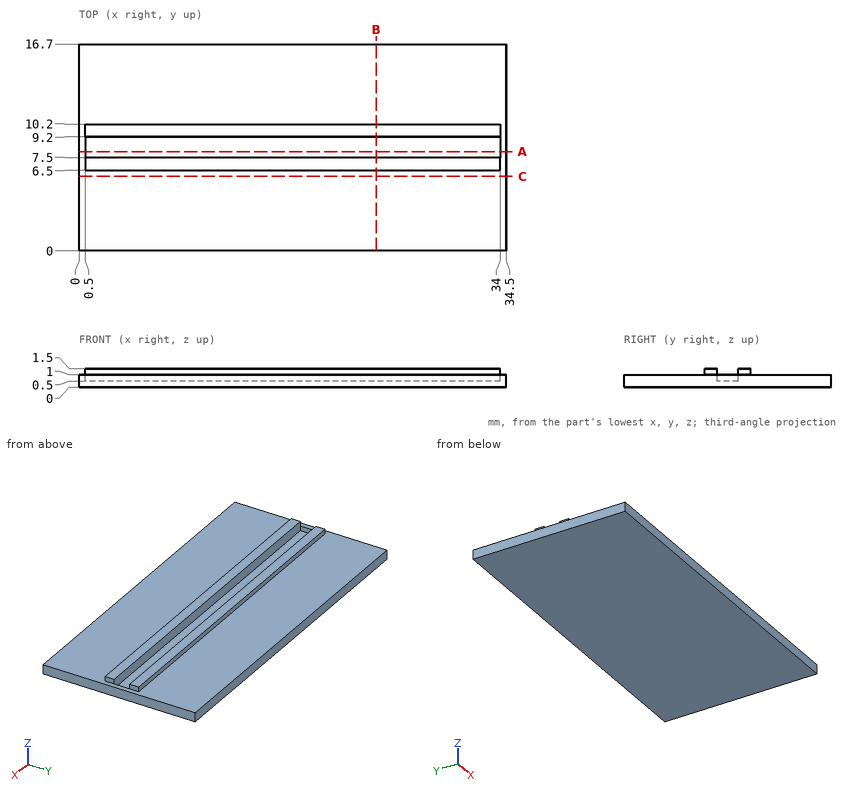
Geometry: see drawing. Coordinates: mm, zero at the bounding-box minimum. Coordinates: 2 decimals unless noted, no trailing zeros. Loops run counter-clockwise (first coordinate to the right, second up) from the corner with the lowest first, then second, coordinate; pieces in that order, holes last. Notation, with made-up numbers: (18, -22.5) - (44, -22.5) arc R23 ccw to (44, -13.5) - close; hole circle Ø4 at (49.25, 55). An arc over 180 degrees is marked (long way). Answer as CSV lines item,"result".
1. Ray query, line 1 (Y direction, x = 31, z = 1.25); line 2 (Y direction, x = 10, z = 0.65); line 3 (Z direction, x = 10, y = 6). Return the intervals inside material, ascending.
Established:
line 1,"y = 6.5 to 7.5, 9.2 to 10.2"
line 2,"y = 0 to 7.5, 9.2 to 16.7"
line 3,"z = 0 to 1"
2. Section A-A (y = 8). Return loops of the section in (x, z).
Established:
outline,"(0, 0) - (34.5, 0) - (34.5, 1) - (34, 1) - (34, 0.5) - (0.5, 0.5) - (0.5, 1) - (0, 1) - close"
3. Section B-B (x = 24). Return loops of the section in (y, z), then the cut area to 4 significant figures.
Established:
outline,"(0, 0) - (16.7, 0) - (16.7, 1) - (10.2, 1) - (10.2, 1.5) - (9.2, 1.5) - (9.2, 0.5) - (7.5, 0.5) - (7.5, 1.5) - (6.5, 1.5) - (6.5, 1) - (0, 1) - close"
area,"16.85 mm2"
4. Section C-C (y = 6). Return loops of the section in (x, z), then the cut area to 3 significant figures.
Established:
outline,"(0, 0) - (34.5, 0) - (34.5, 1) - (0, 1) - close"
area,"34.5 mm2"
5. Contact query for flat-ended pins moving along their axis: pin 1 (0.6 mm diameter, centred on y = 9.5, z = 1.5, fed in from -X); pin 2 (0.8 mm diameter, centred on x = 16.5, y = 8.5, fed in from +Z). Output: stop coordinate, or through.
Established:
pin 1,"stops at x = 0.5"
pin 2,"stops at z = 0.5"
